Check sheet for the modelled part. Datum: model origin and axes. Units: mm. A direction names the side the tool comes from. Give positions to 0.01 mm unless a question says otherwise; leave off trailing zeros. Write each loop counter-clockwise with the first axis right and the second up, starting at its lowest first coordinate (ties: lowest second). Pieces come first, ordered by that corner, then holes. Notation, with made-up numbers: M 62,47 L 103,47 A19 ccw 103,54 Z; hole C -25.5,49 d6. An arc over 180 degrees is marked long. Write item = value, one per line. Start each with the question number.
1) Cross-section at C-C, the plane y = 41.5. Record the cut outline in (x, z).
2) Mould release check, pull along Z, two halves, no side actions. Record for faces 1 (the flat face through (0, 39, 30)), 2 (the cylindrical face through (55.07, 40.24, 32.17)), 3 (the cylindrical face through (55.07, 79.993, 29.34)): released by +Z, released by -Z, zero draft, split by the parting line, or undercut.
3) Scan lines: line 1 along X through (y, z) = (37.5, 15.5); line 2 along Z through (x, y) = (2.25, 50); line 3 along Y through (x, z) = (4, 30). Record each from-to range of solid material in increasing order. Write a range as [from, to].
4) Cross-section at D-D, the plane x = 20. Record the cut outline in (y, z), plus the area to 3 significant figures.
5) Cross-section at B-B, the plane z = 30. Record the cut outline in (x, y).
6) Cross-section at A-A, the plane y = 24.5. Record the cut outline in (x, z).
7) Access from +Z, -Z, +X, -X, +Y, -Y to the whole of each face (thin tool, end or side, straight path). Record for faces 4 (the flat face through (10, 37, 30)), 5 (the flat face through (30, 0, 30)).
8) Go/stop test with flat-tipped pins: pin 1 (12 mm diameter, centred on y = 66.5, z = 53.5, fed in from -X); pin 2 (16 mm diameter, centred on y = 50, z = 30, fed in from +X); pin 3 (8 mm diameter, centred on x = 53, y = 66.5, fed in from -Z); pin 4 (1.5 mm diameter, centred on x = 50.5, z = 25, fed in from +Y). Record where each tip stops, or that it passes through.
```python
from build123d import *

# Parameters (mm, degrees)
EXTRUDE_1_DEPTH     = 60
SKETCH_3_R          = 10
CUT_EXTRUDE_1_DEPTH = 99.488578018
EXTRUDE_START       = 60
SKETCH_8_R          = 30
SKETCH_8_R_2        = 10
EXTRUDE_5_DEPTH     = 60
SKETCH_10_W         = 40
SKETCH_10_H         = 70
CUT_EXTRUDE_3_DEPTH = 60


with BuildPart() as part:
    # 草圖2 → 填料-伸長1 (new body)
    with BuildSketch(Plane.XY):
        Polygon((0, 0), (60, 0), (60, 50), (50, 50), (50, 10), (10, 10), (10, 50), (0, 50), align=None)
    extrude(amount=EXTRUDE_1_DEPTH)

    # 草圖3 → 除料-伸長1 (cut, through all)
    with BuildSketch(Plane(origin=(60, 0, 0), x_dir=(0, 0, -1), z_dir=(1, 0, 0))):
        with Locations((-30, 50)):
            Circle(SKETCH_3_R)
    extrude(amount=-CUT_EXTRUDE_1_DEPTH, mode=Mode.SUBTRACT)

    # 草圖8 → 填料-伸長5 (add)
    with BuildSketch(Plane(origin=(0, 0, 0), x_dir=(0, 0, -1), z_dir=(1, 0, 0)).offset(EXTRUDE_START)):
        with Locations(Location((-30, 50, 0), (0, 0, 180))):
            Circle(SKETCH_8_R)
        with Locations((-30, 50)):
            Circle(SKETCH_8_R_2, mode=Mode.SUBTRACT)
    extrude(amount=-EXTRUDE_5_DEPTH)

    # 草圖10 → 除料-伸長3 (cut)
    with BuildSketch(Plane.XY.offset(60)):
        with Locations((30, 45)):
            Rectangle(SKETCH_10_W, SKETCH_10_H)
    extrude(amount=-CUT_EXTRUDE_3_DEPTH, mode=Mode.SUBTRACT)


solid = part.part
```
Reply:
q1.outline = M 0,0 L 10,0 L 10,24.73 L 0,24.73 Z; M 0,35.27 L 10,35.27 L 10,60 L 0,60 Z; M 50,0 L 60,0 L 60,24.73 L 50,24.73 Z; M 50,35.27 L 60,35.27 L 60,60 L 50,60 Z
q2.face_1 = zero draft
q2.face_2 = undercut
q2.face_3 = split by the parting line
q3.line_1 = [0, 10], [50, 60]
q3.line_2 = [0, 20], [40, 60]
q3.line_3 = [0, 40], [60, 80]
q4.outline = M 0,0 L 10,0 L 10,60 L 0,60 Z
q4.area = 600 mm2
q5.outline = M 0,0 L 60,0 L 60,40 L 50,40 L 50,10 L 10,10 L 10,40 L 0,40 Z; M 0,60 L 10,60 L 10,80 L 0,80 Z; M 50,60 L 60,60 L 60,80 L 50,80 Z
q6.outline = M 0,0 L 10,0 L 10,60 L 0,60 Z; M 50,0 L 60,0 L 60,60 L 50,60 Z
q7.face_4 = +Z, -Z, +Y
q7.face_5 = +Z, -Z, +X, -X, -Y
q8.pin_1 = 0
q8.pin_2 = through
q8.pin_3 = 2.73
q8.pin_4 = 79.7
